Design review of the part built by this model. Coordinates are the model's own, in mm. Face numbers are marked on the shaded views. A direction names the side the tool comes from. Coordinates: 2 decimals unless noted, no trailing zeros. Write each loop counter-clockwise with the first axis right and the second up, starting at its lowest first coordinate (ties: lowest second). Pieces come first, ordered by that corner, then holes.
Q1. Mouldability with a two-part tool opening along Z and no side actions: class the marked faces 4, 5 and 6 as pulls with the +Z half, pulls with the -Z half, needs draft (parallel to the pull), parting line crosses it, or undercut.
Q2. Take a section at B-B (y = 10). State how many separate pieces and enclosed holes the cut face has, and give its area (3 significant figures).
Q3. Insertion check: pin 1 (2 mm diameter, centred on x = 96, z = -62, fed in from -Y); pin 2 (7 mm diameter, centred on x = 90.55, z = -36.69, fed in from -Y); pin 3 (6 mm diameter, centred on y = 3.5, z = -83.5, fed in from -X); pin 4 (3 mm diameter, centred on x = 90.55, z = -36.69, fed in from -Y). Each pin has a flat end and moves straight along its axis. Give the tip position at first contact, or say it passes through.
Q4. Take a section at A-A (x = 130). Give the boundary of the cut face in (y, z).
Q5. Machinability: for the marked faces 1, 2 and 3, which of the approach directions +Z, -Z, +X, -X, +Y, -Y give a long, thin tool a straight path to every point of the face, cutting with its end or side? Answer none if there is none.
Q6. Take a section at C-C (z = -119). Give the boundary of the cut face in (x, y), and give its area (3 significant figures).
Q7. For probe 1 along Z at (x, y) = (77.5, 13.5); probe 2 along X at (y, z) = (11, -39.5); probe 3 along X at (y, z) = (8.25, -41.5), list the stretches that pass through material, from the lowest coordinate up.
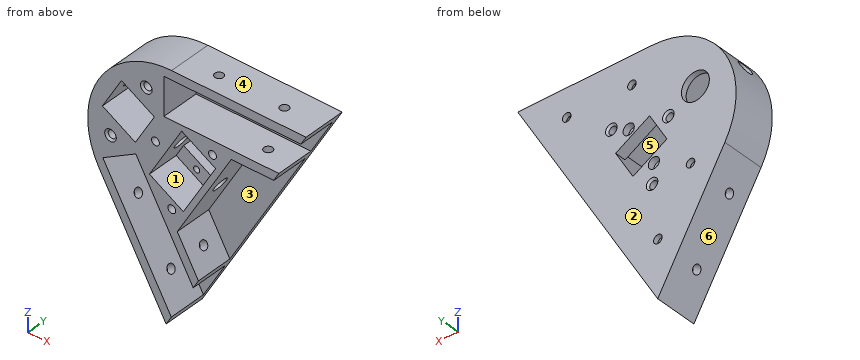
```python
from build123d import *

# Parameters (mm, degrees)
BOSS_EXTRUDE1_DEPTH      = 23
SKETCH2_W                = 100.4
SKETCH2_H                = 20.4
CUT_EXTRUDE2_DEPTH       = 20.4
CUT_EXTRUDE3_DEPTH       = 20
SKETCH7_R                = 2.3
CUT_EXTRUDE6_DEPTH       = 10
SKETCH8_R                = 2.3
CUT_EXTRUDE7_DEPTH       = 10
FILLET3_R                = 45
CUT_EXTRUDE11_DEPTH      = 200.759855827
CUT_EXTRUDE11_DEPTH_BACK = 200.759855827
CUT_EXTRUDE10_DEPTH      = 20
SKETCH32_R               = 2.3
CUT_EXTRUDE18_DEPTH      = 10
SKETCH33_R               = 2.3
CUT_EXTRUDE19_DEPTH      = 10
SKETCH34_R               = 2.3
CUT_EXTRUDE20_DEPTH      = 149.465956609
SKETCH35_R               = 4
CUT_EXTRUDE21_DEPTH      = 152.333845776
SKETCH36_R               = 2.1
CUT_EXTRUDE22_DEPTH      = 200.759855838
SKETCH38_R               = 2.3
CUT_EXTRUDE24_DEPTH      = 10
BOSS_EXTRUDE2_DEPTH      = 6
SKETCH40_R               = 1.65
CUT_EXTRUDE25_DEPTH      = 200.158228561
SKETCH41_R               = 3
CUT_EXTRUDE26_DEPTH      = 3.5
SKETCH42_R               = 2.1
CUT_EXTRUDE27_DEPTH      = 200.759855838
CHAMFER2_SIZE            = 1
SKETCH43_R               = 2.1
CUT_EXTRUDE28_DEPTH      = 15
CHAMFER3_SIZE            = 1
SKETCH45_R               = 2.3
CUT_EXTRUDE29_DEPTH      = 130.123625221
SKETCH46_R               = 4
CUT_EXTRUDE30_DEPTH      = 127.307236488
SKETCH47_R               = 7.5
CUT_EXTRUDE31_DEPTH      = 10


with BuildPart() as part:
    # Sketch1 → Boss-Extrude1 (new body)
    with BuildSketch(Plane(origin=(0, 0, 0), x_dir=(1, 0, 0), z_dir=(0, 1, 0))):
        Polygon((0, 0), (150, 0), (75, 129.903810568), align=None)
    extrude(amount=BOSS_EXTRUDE1_DEPTH)

    # Sketch2 → Cut-Extrude2 (cut)
    with BuildSketch(Plane(origin=(0, 0, 0), x_dir=(1, 0, 0), z_dir=(0, 1, 0))):
        Polygon((108.923840175, 138.261625339), (58.723840175, 51.312674799), (41.056921938, 61.512674799), (91.256921938, 148.461625339), align=None)
        with Locations((124, 15)):
            Rectangle(SKETCH2_W, SKETCH2_H)
    extrude(amount=CUT_EXTRUDE2_DEPTH, mode=Mode.SUBTRACT)

    # Sketch4 → Cut-Extrude3 (cut)
    with BuildSketch(Plane(origin=(0, 0, 0), x_dir=(1, 0, 0), z_dir=(0, 1, 0))):
        Polygon((58.515583945, 45.561933634), (40.848665708, 35.361933634), (51.048665708, 17.695015397), (68.715583945, 27.895015397), align=None)
    extrude(amount=CUT_EXTRUDE3_DEPTH, mode=Mode.SUBTRACT)

    # Sketch7 → Cut-Extrude6 (cut)
    with BuildSketch(Plane(origin=(0, 0, 0), x_dir=(-0.4999999999999978, 0, 0.86602540378444), z_dir=(-0.86602540378444, 0, -0.4999999999999978))):
        with Locations((-130, 10)):
            Circle(SKETCH7_R)
        with Locations((-95, 10)):
            Circle(SKETCH7_R)
    extrude(amount=-CUT_EXTRUDE6_DEPTH, mode=Mode.SUBTRACT)

    # Sketch8 → Cut-Extrude7 (cut)
    with BuildSketch(Plane.XY):
        with Locations((130, 10)):
            Circle(SKETCH8_R)
        with Locations((95, 10)):
            Circle(SKETCH8_R)
    extrude(amount=-CUT_EXTRUDE7_DEPTH, mode=Mode.SUBTRACT)

    # Fillet3
    fillet3_edges = [part.edges().sort_by_distance(p)[0] for p in [
        (0, 11.5, 0),
    ]]
    fillet(fillet3_edges, radius=FILLET3_R)

    # Sketch22 → Cut-Extrude11 (cut, two sides: drawn at the far end of the back side and taken through both)
    with BuildSketch(Plane.XZ.offset(-CUT_EXTRUDE11_DEPTH_BACK)):
        Polygon((83.35335133, -28.147760515), (66.05335133, -58.112239485), (84.23988481, -68.612239485), (101.53988481, -38.647760515), align=None)
    extrude(amount=CUT_EXTRUDE11_DEPTH + CUT_EXTRUDE11_DEPTH_BACK, mode=Mode.SUBTRACT)

    # Sketch21 → Cut-Extrude10 (cut)
    with BuildSketch(Plane.XZ):
        Polygon((132.679491924, -30), (109.996773286, -30), (80.979148757, -80.26), (92.320508076, -99.903810568), align=None)
    extrude(amount=-CUT_EXTRUDE10_DEPTH, mode=Mode.SUBTRACT)

    # Sketch32 → Cut-Extrude18 (cut)
    with BuildSketch(Plane(origin=(0, 0, -30), x_dir=(-1, 0, 0), z_dir=(0, 0, -1))):
        with Locations((-121.338132605, 10)):
            Circle(SKETCH32_R)
    extrude(amount=-CUT_EXTRUDE18_DEPTH, mode=Mode.SUBTRACT)

    # Sketch33 → Cut-Extrude19 (cut)
    with BuildSketch(Plane(origin=(25.980762114, 0, 15), x_dir=(0.4999999999999997, 0, -0.8660254037844388), z_dir=(0.8660254037844389, 0, 0.49999999999999983))):
        with Locations((121.338132605, 10)):
            Circle(SKETCH33_R)
    extrude(amount=-CUT_EXTRUDE19_DEPTH, mode=Mode.SUBTRACT)

    # Sketch34 → Cut-Extrude20 (cut, through all)
    with BuildSketch(Plane(origin=(45.948665708, 0, -26.528474516), x_dir=(-0.5000000000000001, 0, -0.8660254037844386), z_dir=(0.8660254037844386, 0, -0.5000000000000001))):
        with Locations((0, 10)):
            Circle(SKETCH34_R)
    extrude(amount=-CUT_EXTRUDE20_DEPTH, mode=Mode.SUBTRACT)

    # Sketch35 → Cut-Extrude21 (cut, through all)
    with BuildSketch(Plane(origin=(43.350589497, 0, -25.028474516), x_dir=(-0.5000000000000001, 0, -0.8660254037844386), z_dir=(0.8660254037844386, 0, -0.5000000000000001))):
        with Locations((0, 10)):
            Circle(SKETCH35_R)
    extrude(amount=-CUT_EXTRUDE21_DEPTH, mode=Mode.SUBTRACT)

    # Sketch36 → Cut-Extrude22 (cut, through all)
    with BuildSketch(Plane(origin=(0, 23, 0), x_dir=(1, 0, 0), z_dir=(0, 1, 0))):
        with Locations(Location((69.282032303, 40, 0), (0, 0, 270))):
            Circle(SKETCH36_R)
    extrude(amount=-CUT_EXTRUDE22_DEPTH, mode=Mode.SUBTRACT)

    # Sketch38 → Cut-Extrude24 (cut)
    with BuildSketch(Plane.XZ.offset(-20.4)):
        with Locations(Location((88.8, -15, 0), (0, 0, 270))):
            Circle(SKETCH38_R)
        with Locations(Location((123.8, -15, 0), (0, 0, 270))):
            Circle(SKETCH38_R)
        with Locations(Location((57.390381057, -69.403055856, 0), (0, 0, 270))):
            Circle(SKETCH38_R)
        with Locations(Location((74.890381057, -99.713944989, 0), (0, 0, 270))):
            Circle(SKETCH38_R)
    extrude(amount=-CUT_EXTRUDE24_DEPTH, mode=Mode.SUBTRACT)

    # Sketch39 → Boss-Extrude2 (add)
    with BuildSketch(Plane(origin=(0, 23, 0), x_dir=(1, 0, 0), z_dir=(0, 1, 0))):
        Polygon((66.05335133, 58.112239485), (84.23988481, 68.612239485), (88.23988481, 61.684036255), (70.05335133, 51.184036255), align=None)
        Polygon((101.53988481, 38.647760515), (83.35335133, 28.147760515), (79.35335133, 35.075963745), (97.53988481, 45.575963745), align=None)
    extrude(amount=-BOSS_EXTRUDE2_DEPTH)

    # Sketch40 → Cut-Extrude25 (cut, through all)
    with BuildSketch(Plane.XZ.offset(-17)):
        with Locations(Location((90.54661807, -36.688657049, 0), (0, 0, 270))):
            Circle(SKETCH40_R)
        with Locations(Location((77.04661807, -60.071342951, 0), (0, 0, 270))):
            Circle(SKETCH40_R)
    extrude(amount=-CUT_EXTRUDE25_DEPTH, mode=Mode.SUBTRACT)

    # Sketch41 → Cut-Extrude26 (cut)
    with BuildSketch(Plane(origin=(0, 23, 0), x_dir=(1, 0, 0), z_dir=(0, 1, 0))):
        with Locations(Location((77.04661807, 60.071342951, 0), (0, 0, 270))):
            Circle(SKETCH41_R)
        with Locations(Location((90.54661807, 36.688657049, 0), (0, 0, 270))):
            Circle(SKETCH41_R)
    extrude(amount=-CUT_EXTRUDE26_DEPTH, mode=Mode.SUBTRACT)

    # Sketch42 → Cut-Extrude27 (cut, through all)
    with BuildSketch(Plane(origin=(0, 23, 0), x_dir=(1, 0, 0), z_dir=(0, 1, 0))):
        with Locations(Location((99.860934211, 32.446784409, 0), (0, 0, 270))):
            Circle(SKETCH42_R)
        with Locations(Location((78.030206675, 70.258713668, 0), (0, 0, 270))):
            Circle(SKETCH42_R)
    extrude(amount=-CUT_EXTRUDE27_DEPTH, mode=Mode.SUBTRACT)

    # Chamfer2
    chamfer2_edges = [part.edges().sort_by_distance(p)[0] for p in [
        (69.282032303, 23, -42.1),
        (99.860934211, 23, -34.546784409),
        (78.030206675, 23, -72.358713668),
    ]]
    chamfer(chamfer2_edges, length=CHAMFER2_SIZE)

    # Sketch43 → Cut-Extrude28 (cut)
    with BuildSketch(Plane.XZ):
        with Locations(Location((64.382124827, -15.000786763, 0), (0, 0, 270))):
            Circle(SKETCH43_R)
        with Locations(Location((45.182124827, -48.256162268, 0), (0, 0, 270))):
            Circle(SKETCH43_R)
    extrude(amount=-CUT_EXTRUDE28_DEPTH, mode=Mode.SUBTRACT)

    # Chamfer3
    chamfer3_edges = [part.edges().sort_by_distance(p)[0] for p in [
        (64.382124827, 0, -12.900786763),
        (45.182124827, 0, -46.156162268),
    ]]
    chamfer(chamfer3_edges, length=CHAMFER3_SIZE)

    # Sketch45 → Cut-Extrude29 (cut, through all)
    with BuildSketch(Plane(origin=(63.615583945, 0, -36.728474516), x_dir=(0.5, 0, 0.8660254037844386), z_dir=(-0.8660254037844387, 0, 0.5000000000000001))):
        with Locations(Location((0, 10, 0), (0, 0, 180))):
            Circle(SKETCH45_R)
    extrude(amount=-CUT_EXTRUDE29_DEPTH, mode=Mode.SUBTRACT)

    # Sketch46 → Cut-Extrude30 (cut, through all)
    with BuildSketch(Plane(origin=(66.213660157, 0, -38.228474516), x_dir=(0.5, 0, 0.8660254037844386), z_dir=(-0.8660254037844387, 0, 0.5000000000000001))):
        with Locations(Location((0, 10, 0), (0, 0, 180))):
            Circle(SKETCH46_R)
    extrude(amount=-CUT_EXTRUDE30_DEPTH, mode=Mode.SUBTRACT)

    # Sketch47 → Cut-Extrude31 (cut)
    with BuildSketch(Plane.XZ.offset(-20)):
        with Locations(Location((54.782124827, -31.628474516, 0), (0, 0, 270))):
            Circle(SKETCH47_R)
    extrude(amount=-CUT_EXTRUDE31_DEPTH, mode=Mode.SUBTRACT)


solid = part.part
```
Response:
1. face 4: pulls with the +Z half
1. face 5: undercut
1. face 6: pulls with the -Z half
2. separate pieces: 8
2. enclosed holes: 4
2. area: 2,740 mm2
3. pin 1: stops at y = 20
3. pin 2: stops at y = 17
3. pin 3: stops at x = 46.48
3. pin 4: passes through
4. outline: (0, -30) - (20, -30) - (20, -34.64) - (23, -34.64) - (23, 0) - (12.3, 0) - (12.3, -4.8) - (20.4, -4.8) - (20.4, -25.2) - (0, -25.2) - close; (0, -4.8) - (7.7, -4.8) - (7.7, 0) - (0, 0) - close
5. face 1: -Y
5. face 2: +Z, -Z, +X, -X, +Y
5. face 3: +X, -Y
6. outline: (68.7, 0) - (74.25, 0) - (74.25, 20.4) - (81.3, 20.4) - (81.3, 23) - (68.7, 23) - close
6. area: 146 mm2
7. probe 1: z = -125.57 to -124.63, -83.83 to -72.29, -68.23 to -64.72, -38.29 to -25.2, -4.8 to 0
7. probe 2: x = 33.28 to 48.02, 62.02 to 64.27, 76.16 to 76.8, 101.05 to 104.51
7. probe 3: x = 33.08 to 51.48, 60.86 to 64.69, 99.89 to 103.36
